Job drawing, mm, ordinate dimensions from the low corner. One solid piece. Give positions to 0.01 mm unless a question says otherwise; leave off trailing zeros. Loops run counter-clockwise (first coordinate to the right, second up) from the corner with the lowest first, then second, coordinate; pieces in that order, holes last. Notation, with made-up numbers: (19.5, -9) - (66.5, -9) arc R14 cw to (66.5, -5) - close; hole circle Ø9 at (68.5, 46). An arc over 180 degrees is marked (long way). Use a Markdown table: item, result.
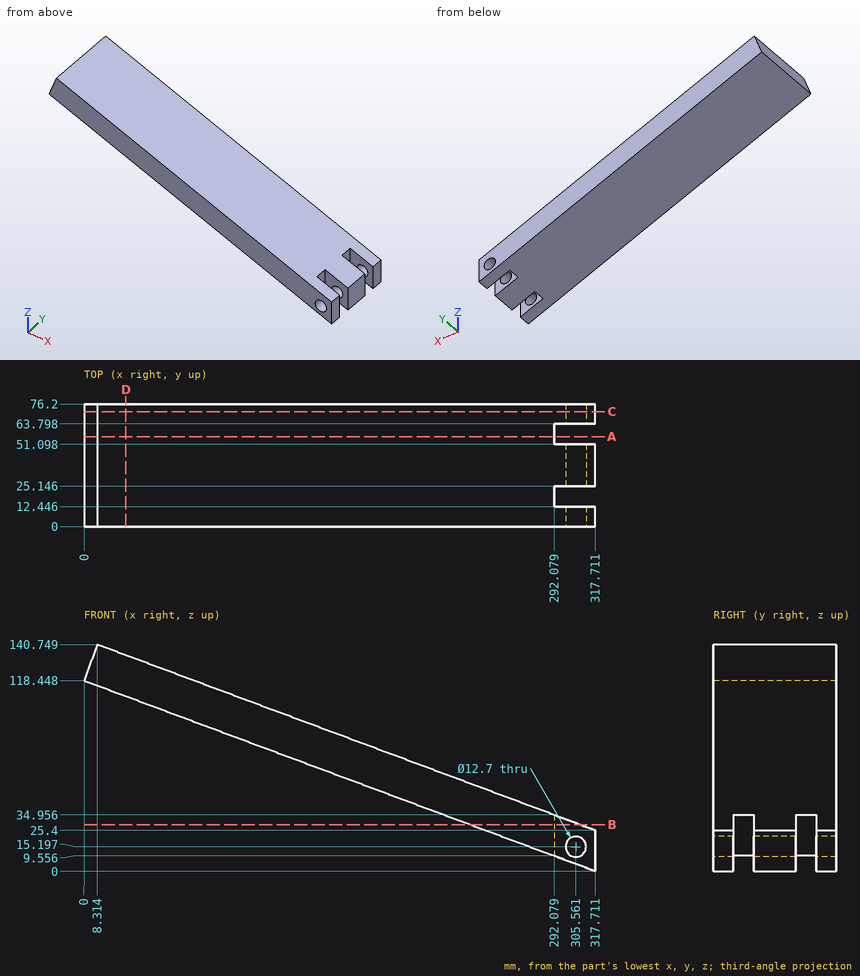
(1) Slice it at C-C, the plane y = 71.5. Write the cut outline in (x, z).
Computed:
| item | result |
|---|---|
| outline | (0, 118.45) - (317.71, 0) - (317.71, 25.4) - (8.31, 140.75) - close; hole circle Ø12.7 at (305.56, 15.2) |
(2) Drill centre lines: probe 1 along Z at (x, y) = (301.5, 69.5) (1 decimal); probe 2 along Z at (x, y) = (147, 24.5) (1 decimal); probe 3 along Z at (x, y) = (166.5, 44.5) (1 decimal). Where is each one in solid material? Low to high. Write a range as [from, to].
Computed:
| item | result |
|---|---|
| probe 1 | [6, 10.3], [20.1, 31.4] |
| probe 2 | [63.6, 89] |
| probe 3 | [56.4, 81.8] |
(3) Slice it at A-A, the plane y = 56. Write the cut outline in (x, z), plus the area to 3 significant figures.
Computed:
| item | result |
|---|---|
| outline | (0, 118.45) - (292.08, 9.56) - (292.08, 34.96) - (8.31, 140.75) - close |
| area | 7,310 mm² |
(4) Slice it at B-B, the plane z = 29. Write the cut outline in (x, y) (1 decimal), plus the area to 3 significant figures.
Computed:
| item | result |
|---|---|
| outline | (239.9, 0) - (308.1, 0) - (308.1, 12.4) - (292.1, 12.4) - (292.1, 25.1) - (308.1, 25.1) - (308.1, 51.1) - (292.1, 51.1) - (292.1, 63.8) - (308.1, 63.8) - (308.1, 76.2) - (239.9, 76.2) - close |
| area | 4,790 mm² |
(5) Pin check, flat tips, straight feed: P1, Ø7.5, axis at x = 303.5, z = 18.5, coming from the -Y side; P2, Ø3, axis at x = 83, y = 49.5, coming from the -Z side (1 decimal); P3, Ø3, axis at x = 236.5, y = 35.5, coming from the +Z side; P4, Ø4, axis at x = 76.5, y = 44.5, coming from the -Z side. Stop position of each tip, or through.
Computed:
| item | result |
|---|---|
| P1 | y = 0 |
| P2 | z = 86.9 |
| P3 | z = 56.24 |
| P4 | z = 89.18 |
(6) Slice it at D-D, the plane x = 26. Write the cut outline in (y, z) (1 decimal).
Computed:
| item | result |
|---|---|
| outline | (0, 108.8) - (76.2, 108.8) - (76.2, 134.2) - (0, 134.2) - close |
